Design review of the part built by this model. Coordinates are the model's own, in mm. Face numbers are marked on the shaded views. A direction names the side the tool comes from. Round coordinates to 2 decimals unless told otherwise and drop trailing zeros. Loops run counter-clockwise (first coordinate to the right, second up) from the corner with the lowest first, then second, coordinate; pieces in that order, holes last. Notation, with made-up numbers: (55, 30.25) - (107, 30.25) arc R22 ccw to (107, 53.25) - close; hole circle Ø10 at (-16, 35.25). An arc over 180 degrees is marked (long way). Answer as CSV lines item,"result". Start each with the question number.
(1) For P1, Ø4, axis at y = -33, z = 18.5, coming from the +X side; P2, Ø3.5, axis at x = 0, z = 19.05, coming from the -Y side, all flat-tipped, find the tip position at first contact; note any pin that passes through.
(2) Consider section B-B (y = -6). Give the boundary of the cut face in (x, z), and give its area (3 significant figures).
(3) For the marked faces 4 and 5, list the 3-axis set-ups (+Z, -Z, +X, -X, +Y, -Y) from which the entire face can be reached by the end or side of a thin tool; tool diameter is ignored.
(4) Consider section A-A (x = 5.25). Give the boundary of the cut face in (y, z).
(5) Mouldability with a two-part tool opening along Y and no side actions: class the marked faces 1, 2 and 3 as released by +Y, released by -Y, zero draft, split by the parting line, or undercut.
(6) Wall thickness on L1, parallel to Y at x = 6, z = 19; L2, parallel to X at y = -58.25, z = 19.05; L3, parallel to X at y = 14.5, z = 33: over which ranges is each line inside the solid? List them lowest first.
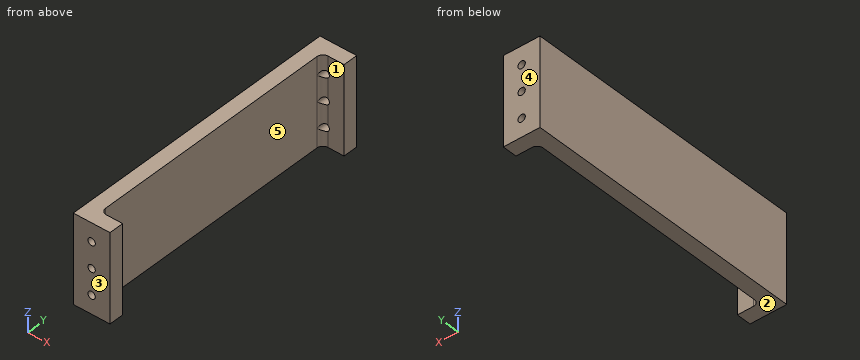
from build123d import *

# Parameters (mm, degrees)
BOSS_EXTRUDE1_DEPTH = 38.1
SKETCH2_R           = 1.5875
CUT_EXTRUDE1_DEPTH  = 130.796935754
FILLET2_R           = 2.54


with BuildPart() as part:
    # Sketch1 → Boss-Extrude1 (new body)
    with BuildSketch(Plane.XY):
        Polygon((-7.9375, -61.9125), (7.9375, -61.9125), (7.9375, -55.5625), (-1.5875, -55.5625), (-1.5875, 55.5625), (7.9375, 55.5625), (7.9375, 61.9125), (-7.9375, 61.9125), align=None)
    extrude(amount=BOSS_EXTRUDE1_DEPTH)

    # Sketch2 → Cut-Extrude1 (cut, through all)
    with BuildSketch(Plane(origin=(0, 61.9125, 0), x_dir=(1, 0, 0), z_dir=(0, 1, 0))):
        with Locations(Location((0, -7.9375, 0), (0, 0, 270))):
            Circle(SKETCH2_R)
        with Locations(Location((0, -19.05, 0), (0, 0, 270))):
            Circle(SKETCH2_R)
        with Locations(Location((0, -30.1625, 0), (0, 0, 270))):
            Circle(SKETCH2_R)
    extrude(amount=-CUT_EXTRUDE1_DEPTH, mode=Mode.SUBTRACT)

    # Fillet2
    # the kernel refuses this fillet: 2.54 mm, written as the material it adds along each edge
    with BuildSketch(Plane(origin=(-1.5875, 55.5625, 30.1625), x_dir=(0, -1, 0), z_dir=(0, 0, 1))) as fillet2_piece_1_section:
        with BuildLine():
            CenterArc((FILLET2_R, FILLET2_R), FILLET2_R, 180, 90)
            Line((0, FILLET2_R), (0, 0))
            Line((0, 0), (FILLET2_R, 0))
        make_face()
    fillet2_piece_1 = extrude(amount=7.9375, mode=Mode.PRIVATE)
    fillet2_piece_1 = fillet2_piece_1 - Plane(origin=(0, 54.97769338, 30.1625), x_dir=(0, 0, 1), z_dir=(0, 1, 0)) * Cylinder(1.5875, 27, mode=Mode.PRIVATE)
    add(fillet2_piece_1)
    with BuildSketch(Plane(origin=(-1.5875, -55.5625, 30.1625), x_dir=(1, 0, 0), z_dir=(0, 0, 1))) as fillet2_piece_2_section:
        with BuildLine():
            CenterArc((FILLET2_R, FILLET2_R), FILLET2_R, 180, 90)
            Line((0, FILLET2_R), (0, 0))
            Line((0, 0), (FILLET2_R, 0))
        make_face()
    fillet2_piece_2 = extrude(amount=7.9375, mode=Mode.PRIVATE)
    fillet2_piece_2 = fillet2_piece_2 - Plane(origin=(0, -54.977693276, 30.1625), x_dir=(0, 0, 1), z_dir=(0, 1, 0)) * Cylinder(1.5875, 27, mode=Mode.PRIVATE)
    add(fillet2_piece_2)
    with BuildSketch(Plane(origin=(-1.5875, 55.5625, 19.05), x_dir=(0, -1, 0), z_dir=(0, 0, 1))) as fillet2_piece_3_section:
        with BuildLine():
            CenterArc((FILLET2_R, FILLET2_R), FILLET2_R, 180, 90)
            Line((0, FILLET2_R), (0, 0))
            Line((0, 0), (FILLET2_R, 0))
        make_face()
    fillet2_piece_3 = extrude(amount=11.1125, mode=Mode.PRIVATE)
    fillet2_piece_3 = fillet2_piece_3 - Plane(origin=(0, 54.968485011, 30.1625), x_dir=(0, 0, 1), z_dir=(0, 1, 0)) * Cylinder(1.5875, 33, mode=Mode.PRIVATE)
    fillet2_piece_3 = fillet2_piece_3 - Plane(origin=(0, 54.968485011, 19.05), x_dir=(0, 0, 1), z_dir=(0, 1, 0)) * Cylinder(1.5875, 33, mode=Mode.PRIVATE)
    add(fillet2_piece_3)
    with BuildSketch(Plane(origin=(-1.5875, 55.5625, 7.9375), x_dir=(0, -1, 0), z_dir=(0, 0, 1))) as fillet2_piece_4_section:
        with BuildLine():
            CenterArc((FILLET2_R, FILLET2_R), FILLET2_R, 180, 90)
            Line((0, FILLET2_R), (0, 0))
            Line((0, 0), (FILLET2_R, 0))
        make_face()
    fillet2_piece_4 = extrude(amount=11.1125, mode=Mode.PRIVATE)
    fillet2_piece_4 = fillet2_piece_4 - Plane(origin=(0, 54.968485011, 19.05), x_dir=(0, 0, 1), z_dir=(0, 1, 0)) * Cylinder(1.5875, 33, mode=Mode.PRIVATE)
    fillet2_piece_4 = fillet2_piece_4 - Plane(origin=(0, 54.968485011, 7.9375), x_dir=(0, 0, 1), z_dir=(0, 1, 0)) * Cylinder(1.5875, 33, mode=Mode.PRIVATE)
    add(fillet2_piece_4)
    with BuildSketch(Plane(origin=(-1.5875, 55.5625, 0), x_dir=(0, -1, 0), z_dir=(0, 0, 1))) as fillet2_piece_5_section:
        with BuildLine():
            CenterArc((FILLET2_R, FILLET2_R), FILLET2_R, 180, 90)
            Line((0, FILLET2_R), (0, 0))
            Line((0, 0), (FILLET2_R, 0))
        make_face()
    fillet2_piece_5 = extrude(amount=7.9375, mode=Mode.PRIVATE)
    fillet2_piece_5 = fillet2_piece_5 - Plane(origin=(0, 54.977693583, 7.9375), x_dir=(0, 0, 1), z_dir=(0, 1, 0)) * Cylinder(1.5875, 27, mode=Mode.PRIVATE)
    add(fillet2_piece_5)
    with BuildSketch(Plane(origin=(-1.5875, -55.5625, 19.05), x_dir=(1, 0, 0), z_dir=(0, 0, 1))) as fillet2_piece_6_section:
        with BuildLine():
            CenterArc((FILLET2_R, FILLET2_R), FILLET2_R, 180, 90)
            Line((0, FILLET2_R), (0, 0))
            Line((0, 0), (FILLET2_R, 0))
        make_face()
    fillet2_piece_6 = extrude(amount=11.1125, mode=Mode.PRIVATE)
    fillet2_piece_6 = fillet2_piece_6 - Plane(origin=(0, -54.968484791, 30.1625), x_dir=(0, 0, 1), z_dir=(0, 1, 0)) * Cylinder(1.5875, 33, mode=Mode.PRIVATE)
    fillet2_piece_6 = fillet2_piece_6 - Plane(origin=(0, -54.968484791, 19.05), x_dir=(0, 0, 1), z_dir=(0, 1, 0)) * Cylinder(1.5875, 33, mode=Mode.PRIVATE)
    add(fillet2_piece_6)
    with BuildSketch(Plane(origin=(-1.5875, -55.5625, 7.9375), x_dir=(1, 0, 0), z_dir=(0, 0, 1))) as fillet2_piece_7_section:
        with BuildLine():
            CenterArc((FILLET2_R, FILLET2_R), FILLET2_R, 180, 90)
            Line((0, FILLET2_R), (0, 0))
            Line((0, 0), (FILLET2_R, 0))
        make_face()
    fillet2_piece_7 = extrude(amount=11.1125, mode=Mode.PRIVATE)
    fillet2_piece_7 = fillet2_piece_7 - Plane(origin=(0, -54.968484789, 19.05), x_dir=(0, 0, 1), z_dir=(0, 1, 0)) * Cylinder(1.5875, 33, mode=Mode.PRIVATE)
    fillet2_piece_7 = fillet2_piece_7 - Plane(origin=(0, -54.968484789, 7.9375), x_dir=(0, 0, 1), z_dir=(0, 1, 0)) * Cylinder(1.5875, 33, mode=Mode.PRIVATE)
    add(fillet2_piece_7)
    with BuildSketch(Plane(origin=(-1.5875, -55.5625, 0), x_dir=(1, 0, 0), z_dir=(0, 0, 1))) as fillet2_piece_8_section:
        with BuildLine():
            CenterArc((FILLET2_R, FILLET2_R), FILLET2_R, 180, 90)
            Line((0, FILLET2_R), (0, 0))
            Line((0, 0), (FILLET2_R, 0))
        make_face()
    fillet2_piece_8 = extrude(amount=7.9375, mode=Mode.PRIVATE)
    fillet2_piece_8 = fillet2_piece_8 - Plane(origin=(0, -54.977693451, 7.9375), x_dir=(0, 0, 1), z_dir=(0, 1, 0)) * Cylinder(1.5875, 27, mode=Mode.PRIVATE)
    add(fillet2_piece_8)


solid = part.part
Determined:
1,P1,"stops at x = -1.59"
1,P2,"stops at y = -61.91"
2,outline,"(-7.94, 0) - (-1.59, 0) - (-1.59, 38.1) - (-7.94, 38.1) - close"
2,area,"242 mm^2"
3,face 4,"+Z, -Z, +X, -X, +Y"
3,face 5,"+Z, -Z, +X"
4,outline,"(-61.91, 0) - (-55.56, 0) - (-55.56, 38.1) - (-61.91, 38.1) - close; (55.56, 0) - (61.91, 0) - (61.91, 38.1) - (55.56, 38.1) - close"
5,face 1,"undercut"
5,face 2,"zero draft"
5,face 3,"released by -Y"
6,L1,"y = -61.91 to -55.56, 55.56 to 61.91"
6,L2,"x = -7.94 to -1.59, 1.59 to 7.94"
6,L3,"x = -7.94 to -1.59"
